from build123d import *

# Parameters (mm, degrees)
BOSS_EXTRUDE1_DEPTH       = 6.35
FILLET1_R                 = 19.05
SKETCH2_W                 = 33.909
SKETCH2_H                 = 3.175
CUT_EXTRUDE1_DEPTH        = 189.494912836
FILLET2_R                 = 1.5875
FILLET2_OF_MIRROR1_R      = 1.5875
SKETCH3_W                 = 6.35
SKETCH3_H                 = 3.175
CUT_EXTRUDE2_DEPTH        = 189.494912836
SKETCH4_W                 = 38.862
SKETCH4_H                 = 47.879
SKETCH4_W_2               = 40.64
SKETCH4_H_2               = 40.386
CUT_EXTRUDE3_DEPTH        = 189.494912836
FILLET3_R                 = 3.175
SKETCH5_W                 = 6.731
SKETCH5_H                 = 25.24125
CUT_EXTRUDE4_DEPTH        = 189.494912836
FILLET4_R                 = 3.175
FILLET5_R                 = 1.5875
F_6_32_TAPPED_HOLE1_D     = 2.7051
F_6_32_TAPPED_HOLE1_DEPTH = 13.335
F_6_32_TAPPED_HOLE1_TIP   = 0.81269403


with BuildPart() as part:
    # Sketch1 → Boss-Extrude1 (new body)
    with BuildSketch(Plane(origin=(0, 0, 0), x_dir=(0, 0, -1), z_dir=(1, 0, 0))):
        Polygon((173.228, 74.041), (173.228, 0), (156.464, 0), (156.464, 46.99), (119.38, 46.99), (119.38, 0), (-119.38, 0), (-119.38, 46.99), (-156.464, 46.99), (-156.464, 0), (-173.228, 0), (-173.228, 74.041), align=None)
    extrude(amount=BOSS_EXTRUDE1_DEPTH)

    # Fillet1
    fillet1_edges = [part.edges().sort_by_distance(p)[0] for p in [
        (3.175, 74.041, 173.228),
        (3.175, 74.041, -173.228),
    ]]
    fillet(fillet1_edges, radius=FILLET1_R)

    # Sketch2 → Cut-Extrude1 (cut, through all)
    with BuildSketch(Plane(origin=(6.35, 0, 0), x_dir=(0, 0, -1), z_dir=(1, 0, 0))):
        with Locations((-137.922, 48.5775)):
            Rectangle(SKETCH2_W, SKETCH2_H)
    cut_extrude1 = extrude(amount=-CUT_EXTRUDE1_DEPTH, mode=Mode.SUBTRACT)

    # Fillet2
    fillet2_edges = [part.edges().sort_by_distance(p)[0] for p in [
        (3.175, 50.165, 154.8765),
        (3.175, 50.165, 120.9675),
    ]]
    fillet(fillet2_edges, radius=FILLET2_R)

    # Mirror1: Cut-Extrude1 across plane
    add(cut_extrude1.mirror(Plane.XY), mode=Mode.SUBTRACT)

    # Fillet2 of Mirror1
    fillet2_of_mirror1_edges = [part.edges().sort_by_distance(p)[0] for p in [
        (3.175, 50.165, -154.8765),
        (3.175, 50.165, -120.9675),
    ]]
    fillet(fillet2_of_mirror1_edges, radius=FILLET2_OF_MIRROR1_R)

    # Sketch3 → Cut-Extrude2 (cut, through all)
    with BuildSketch(Plane(origin=(6.35, 0, 0), x_dir=(0, 0, -1), z_dir=(1, 0, 0))):
        with Locations((-109.855, 1.5875)):
            Rectangle(SKETCH3_W, SKETCH3_H)
        with Locations((-165.989, 1.5875)):
            Rectangle(SKETCH3_W, SKETCH3_H)
    cut_extrude2 = extrude(amount=-CUT_EXTRUDE2_DEPTH, mode=Mode.SUBTRACT)

    # Mirror2: Cut-Extrude2 across plane
    add(cut_extrude2.mirror(Plane.XY), mode=Mode.SUBTRACT)

    # Sketch4 → Cut-Extrude3 (cut, through all)
    with BuildSketch(Plane(origin=(6.35, 0, 0), x_dir=(0, 0, -1), z_dir=(1, 0, 0))):
        with Locations((53.467, 43.7515)):
            Rectangle(SKETCH4_W, SKETCH4_H)
        with Locations((-53.467, 43.7515)):
            Rectangle(SKETCH4_W, SKETCH4_H)
        with Locations((0, 29.718)):
            Rectangle(SKETCH4_W_2, SKETCH4_H_2)
    extrude(amount=-CUT_EXTRUDE3_DEPTH, mode=Mode.SUBTRACT)

    # Fillet3
    fillet3_edges = [part.edges().sort_by_distance(p)[0] for p in [
        (3.175, 19.812, 72.898),
        (3.175, 67.691, 72.898),
        (3.175, 67.691, 34.036),
        (3.175, 19.812, 34.036),
        (3.175, 67.691, -34.036),
        (3.175, 67.691, -72.898),
        (3.175, 19.812, -72.898),
        (3.175, 19.812, -34.036),
        (3.175, 9.525, 20.32),
        (3.175, 49.911, 20.32),
        (3.175, 49.911, -20.32),
        (3.175, 9.525, -20.32),
    ]]
    fillet(fillet3_edges, radius=FILLET3_R)

    # Sketch5 → Cut-Extrude4 (cut, through all)
    with BuildSketch(Plane(origin=(6.35, 0, 0), x_dir=(0, 0, -1), z_dir=(1, 0, 0))):
        with Locations((165.989, 25.320625)):
            Rectangle(SKETCH5_W, SKETCH5_H)
        with Locations((-165.989, 25.320625)):
            Rectangle(SKETCH5_W, SKETCH5_H)
        Polygon((103.124, 12.7), (116.586, 12.7), (114.90325, 37.94125), (104.80675, 37.94125), align=None)
        Polygon((-103.124, 12.7), (-116.586, 12.7), (-114.90325, 37.94125), (-104.80675, 37.94125), align=None)
    extrude(amount=-CUT_EXTRUDE4_DEPTH, mode=Mode.SUBTRACT)

    # Fillet4
    fillet4_edges = [part.edges().sort_by_distance(p)[0] for p in [
        (3.175, 37.94125, -169.3545),
        (3.175, 37.94125, -162.6235),
        (3.175, 37.94125, 169.3545),
        (3.175, 37.94125, 162.6235),
        (3.175, 12.7, -103.124),
        (3.175, 37.94125, -104.80675),
        (3.175, 37.94125, -114.90325),
        (3.175, 12.7, -116.586),
        (3.175, 37.94125, 104.80675),
        (3.175, 12.7, 103.124),
        (3.175, 12.7, 116.586),
        (3.175, 37.94125, 114.90325),
    ]]
    fillet(fillet4_edges, radius=FILLET4_R)

    # Fillet5
    fillet5_edges = [part.edges().sort_by_distance(p)[0] for p in [
        (3.175, 12.7, -169.3545),
        (3.175, 12.7, -162.6235),
        (3.175, 12.7, 169.3545),
        (3.175, 12.7, 162.6235),
    ]]
    fillet(fillet5_edges, radius=FILLET5_R)

    # #6-32 Tapped Hole1
    with Locations(Plane(origin=(3.175, 3.175, 165.989), x_dir=(0, 0, -1), z_dir=(0, -1, 0))):
        with Locations((0, 0), (56.134, 0), (275.844, 0), (331.978, 0)):
            Hole(F_6_32_TAPPED_HOLE1_D / 2, depth=F_6_32_TAPPED_HOLE1_DEPTH)
            with Locations((0, 0, -(F_6_32_TAPPED_HOLE1_DEPTH + F_6_32_TAPPED_HOLE1_TIP / 2))):  # 118° drill point
                Cone(0, F_6_32_TAPPED_HOLE1_D / 2, F_6_32_TAPPED_HOLE1_TIP, mode=Mode.SUBTRACT)


solid = part.part
Can you work these out from the model? Positions are in its coordinate system, mm. A direction names the side the tool comes from. Coordinates: 2 decimals unless noted, no trailing zeros. Loops run counter-clockwise (first coordinate to the right, second up) from the corner with the lowest first, then second, coordinate; pieces in that order, holes last. Notation, with made-up numbers: M 72.25,81.25 L 123.25,81.25 A6 ccw 123.25,88.25 Z; hole C 7,62.5 d5. An arc over 180 degrees is marked long. Return JSON: item names as keys, results as strings. Group by question number.
Item 1: Thinking about a two-plate mould opening in Y: for faces 4 (the flat face through (3, 24, -119.38)), 5 (the flat face through (3, 0, -116)), 6 (the flat face through (3, 19.812, -53)), which applies, released by +Y, released by -Y, zero draft, split by the parting line, or undercut?
Item 2: Imagine slicing it at B-B (z = 150). Please give me the cut outline in (x, y) (3 decimals).
Item 3: Imagine slicing it at A-A (z = -66). Please give me the cut outline in (x, y), and give its area (3 significant figures).
Item 4: On a 3-axis mill with a long thin cutter (end or side, diameter ignored), from which of +Z, -Z, +X, -X, +Y, -Y can I reach the whole of each face in a straight line? I mean faces 1 (the flat face through (5, 3.175, 166)), 2 (the flat face through (3, 43, -72.898)), 3 (the cylindrical face through (3.22, 68.31, -167.8)). Say none if no direction works.
Item 5: I'm going to push flat-ended pins straight in: pin 1 Ø1.9 at (x, z) = (3.5, 166) entering from -Y; pin 2 Ø1.2 at (x, z) = (2, 109) entering from -Y (3 decimals). Where does each tip first touch, or does it pass through?
Item 6: If I drill on L1, parallel to Z at x = 5.5, y = 39; L2, parallel to Z at x = 5.5, y = 3.5; L3, parallel to Z at x = 0.5, y = 48.5, over which ranges is the centre line in solid material (lowest first)? Write a range as from..to.
Verdict:
{
 "1": {"face 4": "zero draft", "face 5": "released by -Y", "face 6": "undercut"},
 "2": {"outline": "M 0,50.165 L 6.35,50.165 L 6.35,74.041 L 0,74.041 Z"},
 "3": {"outline": "M 0,0 L 6.35,0 L 6.35,19.81 L 0,19.81 Z; M 0,67.69 L 6.35,67.69 L 6.35,74.04 L 0,74.04 Z", "area": "166 mm^2"},
 "4": {"face 1": "+X, -X, -Y", "face 2": "+X, -X", "face 3": "-Z, +X, -X, +Y"},
 "5": {"pin 1": "stops at y = 37.85", "pin 2": "stops at y = 3.175"},
 "6": {"L1": "z = -173.23..-156.46, -119.38..-72.9, -34.04..-20.32, 20.32..34.04, 72.9..119.38, 156.46..173.23", "L2": "z = -173.23..-156.46, -119.38..119.38, 156.46..173.23", "L3": "z = -173.23..-154.88, -120.97..-72.9, -34.04..-19.78, 19.78..34.04, 72.9..120.97, 154.88..173.23"}
}
